from build123d import *

# Parameters (mm, degrees)
F0_W        = 258.2719624043
F0_H        = 118.0609464645
F1_DEPTH    = 76.2
F2_R        = 42.468670908
F3_DEPTH    = 25.4
F4_T        = -2.54
F5_R        = 42.5232314901
F6_DEPTH    = 25.4
F7_T        = 2.54
F7_T3_DEPTH = 76.2
F7_T5_DEPTH = 258.2719624043
F7_T7_DEPTH = 118.0609464645
F8_W        = 87.3291939497
F8_H        = 24.8894710094
F9_DEPTH    = 11.938
F10_R       = 5.08
F12_D       = 6.35
F14_D       = 6.35


# Not quite as in the source:
# - a shell that OpenCascade refuses in one call is made with other operations: the cavity is built on its own and cut out


with BuildPart() as f1:
    # F0 (on Front) → F1 (new body)
    with BuildSketch(Plane.XZ):
        Rectangle(F0_W, F0_H)
    extrude(amount=F1_DEPTH)

    # F2 (on face) → F3 (join)
    with BuildSketch(Plane.XZ.offset(76.2)):
        with Locations((-77.9456719756, 0)):
            Circle(F2_R)
    extrude(amount=F3_DEPTH)

    # F4
    f4_openings = [f1.faces().sort_by_distance(p)[0] for p in [
        (-77.945672, -101.6, 0),
    ]]
    offset(amount=F4_T, openings=f4_openings, kind=Kind.INTERSECTION)

    # F5 (on face) → F6 (join)
    with BuildSketch(Plane.XZ.offset(76.2)):
        with Locations((75.858682394, 0)):
            Circle(F5_R)
    extrude(amount=F6_DEPTH)

    # F7: shell of thickness 2.54, made by hand


with BuildPart() as f7_core1:
    # F7_t2: copy of F1
    add(f1.part)

    # the walls: a layer under each face that stays
    f7_faces = [f7_core1.faces().sort_by_distance(p)[0] for p in [
        (0, -38.1, 56.4904732323),
        (126.5959812021, -38.1, 0),
        (0, -73.66, 0),
        (-126.5959812021, -38.1, 0),
        (0, -2.54, 0),
        (0, -38.1, -56.4904732323),
        (-117.8743428837, -87.63, 0),
        (-106.2581192476, -101.6, -28.312447272),
        (-120.4143428837, -88.9, 0),
        (0, -76.2, 0),
        (0, -38.1, 59.0304732323),
        (129.1359812021, -38.1, 0),
        (-129.1359812021, -38.1, 0),
        (0, -38.1, -59.0304732323),
        (33.3354509039, -88.9, 0),
        (0, 0, 0),
    ]]
    thicken(f7_faces, amount=-F7_T, mode=Mode.SUBTRACT)

    # F7_s4 → F7_t3 (cut)
    with BuildSketch(Plane.XZ):
        Polygon((126.5705812021, 56.4650732323), (126.5959812021, 59.0304732323), (129.1359812021, 59.0304732323), (129.1359812021, 56.4904732323), align=None)
        Polygon((-126.5705812021, 56.4650732323), (-126.5959812021, 59.0304732323), (-129.1359812021, 59.0304732323), (-129.1359812021, 56.4904732323), align=None)
        Polygon((126.5705812021, -56.4650732323), (129.1359812021, -56.4904732323), (129.1359812021, -59.0304732323), (126.5959812021, -59.0304732323), align=None)
        Polygon((-126.5705812021, -56.4650732323), (-129.1359812021, -56.4904732323), (-129.1359812021, -59.0304732323), (-126.5959812021, -59.0304732323), align=None)
    extrude(amount=F7_T3_DEPTH, mode=Mode.SUBTRACT)

    # F7_s6 → F7_t5 (cut)
    with BuildSketch(Plane.YZ.offset(-129.1359812021)):
        Polygon((-73.6346, 56.4650732323), (-73.66, 59.0304732323), (-76.2, 59.0304732323), (-76.2, 56.4904732323), align=None)
        Polygon((-2.5654, 56.4650732323), (-2.54, 59.0304732323), (0, 59.0304732323), (0, 56.4904732323), align=None)
        Polygon((-73.6346, -56.4650732323), (-76.2, -56.4904732323), (-76.2, -59.0304732323), (-73.66, -59.0304732323), align=None)
        Polygon((-2.5654, -56.4650732323), (0, -56.4904732323), (0, -59.0304732323), (-2.54, -59.0304732323), align=None)
    extrude(amount=F7_T5_DEPTH, mode=Mode.SUBTRACT)

    # F7_s8 → F7_t7 (cut)
    with BuildSketch(Plane.XY.offset(-59.0304732323)):
        Polygon((126.5705812021, -73.6346), (129.1359812021, -73.66), (129.1359812021, -76.2), (126.5959812021, -76.2), align=None)
        Polygon((126.5705812021, -2.5654), (129.1359812021, -2.54), (129.1359812021, 0), (126.5959812021, 0), align=None)
        Polygon((-126.5705812021, -73.6346), (-126.5959812021, -76.2), (-129.1359812021, -76.2), (-129.1359812021, -73.66), align=None)
        Polygon((-126.5705812021, -2.5654), (-129.1359812021, -2.54), (-129.1359812021, 0), (-126.5959812021, 0), align=None)
    extrude(amount=F7_T7_DEPTH, mode=Mode.SUBTRACT)

    # F7_s9 → F7_t10 (revolve, cut)
    with BuildSketch(Plane.XY):
        Polygon((-35.4516010676, -76.2254), (-38.0170010676, -76.2), (-38.0170010676, -73.66), (-35.4770010676, -73.66), align=None)
    revolve(axis=Axis((-77.9456719756, -76.2, 0), (0, -1, 0)), mode=Mode.SUBTRACT)

    # F7_s11 → F7_t12 (revolve, cut)
    with BuildSketch(Plane.XY):
        Polygon((118.4073138841, -76.2254), (118.3819138841, -73.66), (115.8419138841, -73.66), (115.8419138841, -76.2), align=None)
    revolve(axis=Axis((75.858682394, -76.2, 0), (0, -1, 0)), mode=Mode.SUBTRACT)


with BuildPart() as f1_1:
    add(f1.part)

    # what is left inside the walls is the cavity
    f7_cavity = [f7_core1.part.solids().sort_by_distance(p)[0] for p in [
        (35.900851, -93.133333, 0),
    ]]
    add(f7_cavity, mode=Mode.SUBTRACT)

    # F8 (on face) → F9 (join)
    with BuildSketch(Plane.XY.offset(59.0304732323)):
        with Locations((0, -20.2801432461)):
            Rectangle(F8_W, F8_H)
    extrude(amount=F9_DEPTH)

    # F10
    f10_edges = [f1_1.edges().sort_by_distance(p)[0] for p in [
        (-129.135981, -38.1, 59.030473),
        (-129.135981, -38.1, -59.030473),
        (129.135981, -38.1, 59.030473),
        (129.135981, -38.1, -59.030473),
        (129.135981, -76.2, 0),
        (0, -76.2, 59.030473),
        (0, -76.2, -59.030473),
        (129.135981, 0, 0),
        (0, 0, 59.030473),
        (0, 0, -59.030473),
        (-129.135981, 0, 0),
        (-129.135981, -76.2, 0),
        (-43.664597, -20.280143, 70.968473),
        (0, -32.724879, 70.968473),
        (0, -7.835408, 70.968473),
        (43.664597, -20.280143, 70.968473),
        (-43.664597, -32.724879, 64.999473),
        (-43.664597, -7.835408, 64.999473),
        (43.664597, -32.724879, 64.999473),
        (43.664597, -7.835408, 64.999473),
    ]]
    fillet(f10_edges, radius=F10_R)

    # F12 (through all)
    with Locations(Plane.XZ.offset(76.2)):
        with Locations((-4.5539974235, 40.1396788657)):
            Hole(F12_D / 2)

    # F14 (through all)
    with Locations(Plane.XZ.offset(76.2)):
        with Locations((-37.6857295632, 38.1780304015), (-23.1191907078, 27.56604366), (10.8693959191, 30.9581160545), (33.4332510829, 36.6552881896), (24.007840082, 23.2110135257), (-8.8382726535, 17.2407273203), (5.1570278592, 20.6584427506), (-18.8349168748, 6.6602416337), (14.5824337378, 10.9119648114), (27.149643749, 3.7382091396), (24.007840082, -15.726538375), (14.2968157306, -4.8344726674), (-29.9740321934, -7.9270545393), (-5.6964703836, -10.5349421501), (-23.1191907078, -21.9648182392), (-12.2656933963, -24.5554894209), (-28.8315601647, -34.8412431777), (7.4419751763, -21.1450979114), (18.8667103648, -34.3298055232)):
            Hole(F14_D / 2)


solid = f1_1.part
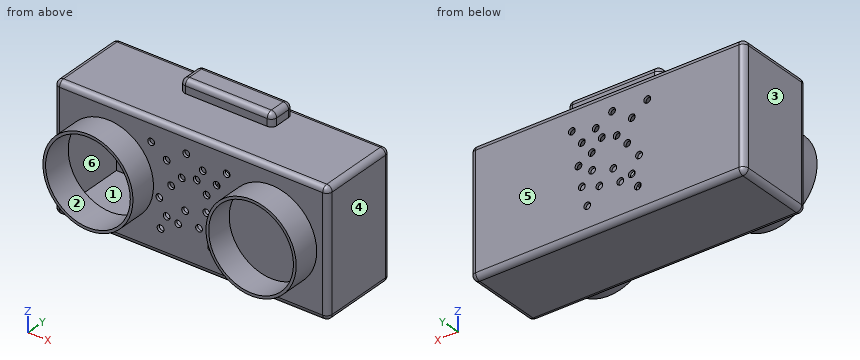
Verification items for the finished model (mm, model axes). Face numbers are marked on the shaded views. A direction names the side the tool comes from. Round coordinates to 2 decimals unless told otherwise and drop trailing zeros. Loops run counter-clockwise (first coordinate to the right, second up) from the corner with the lowest first, then second, coordinate; pieces in that order, holes last. Notation, with made-up numbers: (-16.5, -40) - (23.5, -40) arc R24 cw to (23.5, -20) - close; hole circle Ø9 at (-12, 63.5). An arc over 180 degrees is marked (long way). Use a Markdown table: item, result. Add a question column.
1. Section check B-B, the plane x = 51. Record the boundary of the cut face in (y, z), plus the area to 3 significant figures.
2. Thickness scan on probe 1 along Z at (x, y) = (89, -28); probe 2 along Y at (x, z) = (45, -41); probe 3 along Y at (x, z) = (-41.5, -21.5). Record the ranges inside material, lowest first. Write a range as [from, to].
3. Section check C-C, the plane x = -50.5. Record the boundary of the cut face in (y, z).
4. Section check D-D, the plane x = -88.5. Record the boundary of the cut face in (y, z), plus the area to 3 significant figures.
5. Section check A-A, the plane y = -94.5. Record the boundary of the cut face in (x, z).
6. Gauge pin test, flat ends, axial feed: pin 1 (4 mm diameter, centred on x = -37.69, z = 38.18, fed in from +Y); pin 2 (10 mm diameter, centred on x = 24.01, z = 23.21, fed in from -Y); pin 3 (3 mm diameter, centred on y = -82.5, z = 28.5, fed in from -X). Record the tip position at first contact, or that the pin passes through.
7. Access from +Z, -Z, +X, -X, +Y, -Y to the whole of each face (thin tool, end or side, straight path). Record for the marked faces 1, 2 and 3.
8. Release check for a two-part mould opening along Y. For the marked faces 4, 5 and 6 record: released by +Y, released by -Y, zero draft, split by the parting line, or undercut.
Checks:
| question | item | result |
|---|---|---|
| 1 | outline | (-101.6, -34.5) - (-76.2, -34.5) - (-76.2, -53.95) arc R5.08 ccw to (-71.12, -59.03) - (-5.08, -59.03) arc R5.08 ccw to (0, -53.95) - (0, 53.95) arc R5.08 ccw to (-5.08, 59.03) - (-71.12, 59.03) arc R5.08 ccw to (-76.2, 53.95) - (-76.2, 34.5) - (-101.6, 34.5) - (-101.6, 31.32) - (-76.2, 31.32) - (-76.2, -31.32) - (-101.6, -31.32) - close; hole (-73.66, -56.49) - (-2.54, -56.49) - (-2.54, 56.49) - (-73.66, 56.49) - close |
| 1 | area | 1,100 mm^2 |
| 2 | probe 1 | z = [-59.03, -56.49], [56.49, 59.03] |
| 2 | probe 2 | y = [-76.2, -73.66], [-2.54, 0] |
| 2 | probe 3 | y = [-101.6, -73.66], [-2.54, 0] |
| 3 | outline | (-101.6, -32.41) - (-76.2, -32.41) - (-76.2, -53.95) arc R5.08 ccw to (-71.12, -59.03) - (-5.08, -59.03) arc R5.08 ccw to (0, -53.95) - (0, 53.95) arc R5.08 ccw to (-5.08, 59.03) - (-71.12, 59.03) arc R5.08 ccw to (-76.2, 53.95) - (-76.2, 32.41) - (-101.6, 32.41) - (-101.6, 29) - (-73.66, 29) - (-73.66, 56.49) - (-2.54, 56.49) - (-2.54, -56.49) - (-73.66, -56.49) - (-73.66, -29) - (-101.6, -29) - close |
| 4 | outline | (-101.6, -41.14) - (-76.2, -41.14) - (-76.2, -53.95) arc R5.08 ccw to (-71.12, -59.03) - (-5.08, -59.03) arc R5.08 ccw to (0, -53.95) - (0, 53.95) arc R5.08 ccw to (-5.08, 59.03) - (-71.12, 59.03) arc R5.08 ccw to (-76.2, 53.95) - (-76.2, 41.14) - (-101.6, 41.14) - (-101.6, 38.51) - (-73.66, 38.51) - (-73.66, 56.49) - (-2.54, 56.49) - (-2.54, -56.49) - (-73.66, -56.49) - (-73.66, -38.51) - (-101.6, -38.51) - close |
| 4 | area | 877 mm^2 |
| 5 | outline | circle Ø84.94 at (-77.95, 0); circle Ø85.05 at (75.86, 0); hole circle Ø79.86 at (-77.95, 0); hole circle Ø79.97 at (75.86, 0) |
| 6 | pin 1 | passes through |
| 6 | pin 2 | stops at y = -76.2 |
| 6 | pin 3 | stops at x = -110.73 |
| 7 | face 1 | none |
| 7 | face 2 | -Y |
| 7 | face 3 | +Z, -Z, -X, +Y, -Y |
| 8 | face 4 | zero draft |
| 8 | face 5 | released by +Y |
| 8 | face 6 | undercut |
